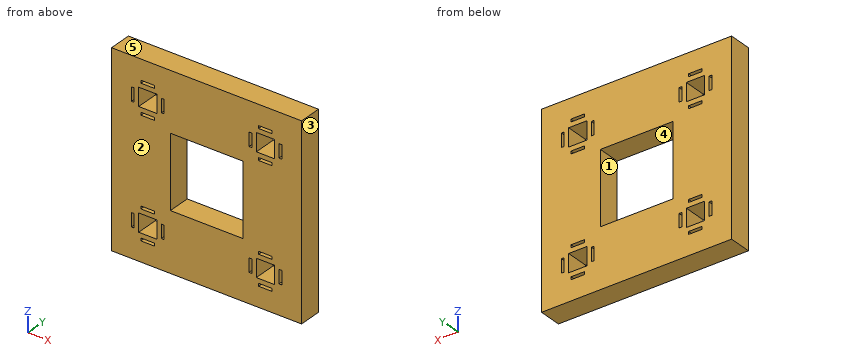
Autodesk Inventor part; units mm, degrees
ref_plane "YZ Plane" through (0, 0, 0) normal (1, 0, 0) x (0, 1, 0)
ref_plane "XZ Plane" through (0, 0, 0) normal (0, 1, 0) x (-1, 0, 0)
ref_plane "XY Plane" through (0, 0, 0) normal (0, 0, 1) x (1, 0, 0)
sketch "Sketch1" plane through (0, 0, 0) normal (0, 0, 1) x (1, 0, 0)
  line L0 (-105, 12.5) -> (105, 12.5)
  line L1 (105, 12.5) -> (105, -12.5)
  line L2 (105, -12.5) -> (-105, -12.5)
  line L3 (-105, -12.5) -> (-105, 12.5)
  line L4 (-105, 12.5) -> (105, -12.5) construction
  line L5 (105, 12.5) -> (-105, -12.5) construction
  point P0 (0, 0)
  dimension "d0" = 210
  dimension "d1" = 25
extrude "Extrusion1" add sketch "Sketch1" along normal mid plane 210
sketch "Sketch2" plane through (-105, -12.5, 105) normal (0, -1, 0) x (1, 0, 0)
  line L0 (0, -210) -> (0, 0)
  line L1 (0, -40) -> (210, -40)
  line L2 (210, -210) -> (210, 0)
  line L3 (0, -170) -> (210, -170)
  line L4 (0, -105) -> (210, -105)
  line L5 (0, 0) -> (210, 0)
  line L6 (105, 0) -> (105, -210)
  line L7 (170, 0) -> (170, -210)
  line L8 (40, 0) -> (40, -210)
  line L9 (210, -210) -> (0, -210)
  line L10 (0, 0) -> (0, -210)
  line L11 (162.5, -21.92) -> (177.5, -21.92)
  line L12 (177.5, -21.92) -> (177.5, -25)
  line L13 (177.5, -25) -> (162.5, -25)
  line L14 (162.5, -25) -> (162.5, -21.92)
  line L15 (162.5, -21.92) -> (177.5, -25) construction
  line L16 (177.5, -21.92) -> (162.5, -25) construction
  line L17 (188.08, -32.5) -> (185, -32.5)
  line L18 (185, -32.5) -> (185, -47.5)
  line L19 (185, -47.5) -> (188.08, -47.5)
  line L20 (188.08, -47.5) -> (188.08, -32.5)
  line L21 (188.08, -32.5) -> (185, -47.5) construction
  line L22 (185, -32.5) -> (188.08, -47.5) construction
  line L23 (162.5, -58.08) -> (177.5, -58.08)
  line L24 (177.5, -58.08) -> (177.5, -55)
  line L25 (177.5, -55) -> (162.5, -55)
  line L26 (162.5, -55) -> (162.5, -58.08)
  line L27 (162.5, -58.08) -> (177.5, -55) construction
  line L28 (177.5, -58.08) -> (162.5, -55) construction
  line L29 (188.08, -47.5) -> (185, -47.5)
  line L30 (185, -47.5) -> (185, -32.5)
  line L31 (185, -32.5) -> (188.08, -32.5)
  line L32 (188.08, -32.5) -> (188.08, -47.5)
  line L33 (188.08, -47.5) -> (185, -32.5) construction
  line L34 (185, -47.5) -> (188.08, -32.5) construction
  line L35 (151.92, -32.5) -> (155, -32.5)
  line L36 (155, -32.5) -> (155, -47.5)
  line L37 (155, -47.5) -> (151.92, -47.5)
  line L38 (151.92, -47.5) -> (151.92, -32.5)
  line L39 (151.92, -32.5) -> (155, -47.5) construction
  line L40 (155, -32.5) -> (151.92, -47.5) construction
  line L41 (155, -32.5) -> (151.92, -32.5)
  line L42 (155, -47.5) -> (155, -32.5)
  line L43 (151.92, -32.5) -> (151.92, -47.5)
  line L44 (155, -47.5) -> (151.92, -32.5) construction
  line L45 (151.92, -47.5) -> (155, -47.5)
  line L46 (151.92, -47.5) -> (155, -32.5) construction
  line L47 (47.5, -21.92) -> (32.5, -21.92)
  line L48 (32.5, -21.92) -> (32.5, -25)
  line L49 (32.5, -25) -> (47.5, -25)
  line L50 (47.5, -25) -> (47.5, -21.92)
  line L51 (47.5, -21.92) -> (32.5, -25) construction
  line L52 (32.5, -21.92) -> (47.5, -25) construction
  line L53 (21.92, -32.5) -> (25, -32.5)
  line L54 (25, -32.5) -> (25, -47.5)
  line L55 (25, -47.5) -> (21.92, -47.5)
  line L56 (21.92, -47.5) -> (21.92, -32.5)
  line L57 (21.92, -32.5) -> (25, -47.5) construction
  line L58 (25, -32.5) -> (21.92, -47.5) construction
  line L59 (32.5, -55) -> (47.5, -55)
  line L60 (47.5, -58.08) -> (32.5, -58.08)
  line L61 (32.5, -58.08) -> (47.5, -55) construction
  line L62 (47.5, -58.08) -> (32.5, -55) construction
  line L63 (47.5, -55) -> (47.5, -58.08)
  line L64 (32.5, -58.08) -> (32.5, -55)
  line L65 (25, -32.5) -> (21.92, -32.5)
  line L66 (25, -47.5) -> (25, -32.5)
  line L67 (21.92, -32.5) -> (21.92, -47.5)
  line L68 (25, -47.5) -> (21.92, -32.5) construction
  line L69 (21.92, -47.5) -> (25, -47.5)
  line L70 (21.92, -47.5) -> (25, -32.5) construction
  line L71 (55, -32.5) -> (58.08, -32.5)
  line L72 (58.08, -32.5) -> (55, -32.5)
  line L73 (55, -47.5) -> (55, -32.5)
  line L74 (55, -32.5) -> (55, -47.5)
  line L75 (58.08, -47.5) -> (55, -47.5)
  line L76 (58.08, -32.5) -> (58.08, -47.5)
  line L77 (55, -47.5) -> (58.08, -32.5) construction
  line L78 (58.08, -47.5) -> (55, -32.5) construction
  line L79 (55, -47.5) -> (58.08, -47.5)
  line L80 (58.08, -47.5) -> (58.08, -32.5)
  line L81 (55, -32.5) -> (58.08, -47.5) construction
  line L82 (58.08, -32.5) -> (55, -47.5) construction
  line L83 (162.5, -188.08) -> (177.5, -188.08)
  line L84 (177.5, -188.08) -> (177.5, -185)
  line L85 (177.5, -185) -> (162.5, -185)
  line L86 (162.5, -185) -> (162.5, -188.08)
  line L87 (162.5, -188.08) -> (177.5, -185) construction
  line L88 (177.5, -188.08) -> (162.5, -185) construction
  line L89 (188.08, -177.5) -> (185, -177.5)
  line L90 (185, -177.5) -> (185, -162.5)
  line L91 (185, -162.5) -> (188.08, -162.5)
  line L92 (188.08, -162.5) -> (188.08, -177.5)
  line L93 (188.08, -177.5) -> (185, -162.5) construction
  line L94 (185, -177.5) -> (188.08, -162.5) construction
  line L95 (177.5, -155) -> (162.5, -155)
  line L96 (162.5, -151.92) -> (177.5, -151.92)
  line L97 (177.5, -151.92) -> (162.5, -155) construction
  line L98 (162.5, -151.92) -> (177.5, -155) construction
  line L99 (162.5, -155) -> (162.5, -151.92)
  line L100 (177.5, -151.92) -> (177.5, -155)
  line L101 (185, -177.5) -> (188.08, -177.5)
  line L102 (185, -162.5) -> (185, -177.5)
  line L103 (188.08, -177.5) -> (188.08, -162.5)
  line L104 (185, -162.5) -> (188.08, -177.5) construction
  line L105 (188.08, -162.5) -> (185, -162.5)
  line L106 (188.08, -162.5) -> (185, -177.5) construction
  line L107 (155, -177.5) -> (151.92, -177.5)
  line L108 (151.92, -177.5) -> (155, -177.5)
  line L109 (155, -162.5) -> (155, -177.5)
  line L110 (155, -177.5) -> (155, -162.5)
  line L111 (151.92, -162.5) -> (155, -162.5)
  line L112 (151.92, -177.5) -> (151.92, -162.5)
  line L113 (155, -162.5) -> (151.92, -177.5) construction
  line L114 (151.92, -162.5) -> (155, -177.5) construction
  line L115 (155, -162.5) -> (151.92, -162.5)
  line L116 (151.92, -162.5) -> (151.92, -177.5)
  line L117 (155, -177.5) -> (151.92, -162.5) construction
  line L118 (151.92, -177.5) -> (155, -162.5) construction
  line L119 (55, -177.5) -> (58.08, -177.5)
  line L120 (58.08, -177.5) -> (58.08, -162.5)
  line L121 (55, -162.5) -> (58.08, -177.5) construction
  line L122 (58.08, -162.5) -> (55, -177.5) construction
  line L123 (58.08, -177.5) -> (55, -177.5)
  line L124 (58.08, -162.5) -> (58.08, -177.5)
  line L125 (55, -177.5) -> (58.08, -162.5) construction
  line L126 (58.08, -177.5) -> (55, -162.5) construction
  line L127 (58.08, -162.5) -> (55, -162.5)
  line L128 (55, -162.5) -> (58.08, -162.5)
  line L129 (25, -162.5) -> (21.92, -162.5)
  line L130 (21.92, -162.5) -> (25, -162.5)
  line L131 (25, -177.5) -> (25, -162.5)
  line L132 (25, -162.5) -> (25, -177.5)
  line L133 (21.92, -162.5) -> (21.92, -177.5)
  line L134 (25, -177.5) -> (21.92, -162.5) construction
  line L135 (21.92, -177.5) -> (25, -162.5) construction
  line L136 (21.92, -177.5) -> (25, -177.5)
  line L137 (21.92, -162.5) -> (25, -177.5) construction
  line L138 (21.92, -177.5) -> (21.92, -162.5)
  line L139 (25, -177.5) -> (21.92, -177.5)
  line L140 (25, -162.5) -> (21.92, -177.5) construction
  line L141 (47.5, -188.08) -> (32.5, -188.08)
  line L142 (32.5, -188.08) -> (32.5, -185)
  line L143 (32.5, -185) -> (47.5, -185)
  line L144 (47.5, -185) -> (47.5, -188.08)
  line L145 (47.5, -188.08) -> (32.5, -185) construction
  line L146 (32.5, -188.08) -> (47.5, -185) construction
  line L147 (55, -162.5) -> (55, -177.5)
  line L148 (55, -177.5) -> (55, -162.5)
  line L149 (32.5, -151.92) -> (32.5, -155)
  line L150 (32.5, -155) -> (47.5, -155)
  line L151 (32.5, -151.92) -> (47.5, -155) construction
  line L152 (47.5, -151.92) -> (32.5, -155) construction
  line L153 (47.5, -155) -> (47.5, -151.92)
  line L154 (47.5, -151.92) -> (32.5, -151.92)
  line L155 (160, -30) -> (180, -30)
  line L156 (180, -30) -> (180, -50)
  line L157 (180, -50) -> (160, -50)
  line L158 (160, -50) -> (160, -30)
  line L159 (160, -30) -> (180, -50) construction
  line L160 (180, -30) -> (160, -50) construction
  line L161 (30, -50) -> (50, -50)
  line L162 (50, -50) -> (50, -30)
  line L163 (50, -30) -> (30, -30)
  line L164 (30, -30) -> (30, -50)
  line L165 (30, -50) -> (50, -30) construction
  line L166 (50, -50) -> (30, -30) construction
  line L167 (30, -160) -> (50, -160)
  line L168 (50, -160) -> (50, -180)
  line L169 (50, -180) -> (30, -180)
  line L170 (30, -180) -> (30, -160)
  line L171 (30, -160) -> (50, -180) construction
  line L172 (50, -160) -> (30, -180) construction
  line L173 (160, -160) -> (180, -160)
  line L174 (180, -160) -> (180, -180)
  line L175 (180, -180) -> (160, -180)
  line L176 (160, -180) -> (160, -160)
  line L177 (160, -160) -> (180, -180) construction
  line L178 (180, -160) -> (160, -180) construction
  point P0 (105, -105)
  point P1 (170, -23.46)
  point P2 (186.54, -40)
  point P3 (170, -56.54)
  point P4 (153.46, -40)
  point P5 (40, -23.46)
  point P6 (23.46, -40)
  point P7 (40, -56.54)
  point P8 (56.54, -40)
  point P9 (170, -186.54)
  point P10 (186.54, -170)
  point P11 (170, -153.46)
  point P12 (153.46, -170)
  point P13 (56.54, -170)
  point P14 (23.46, -170)
  point P15 (40, -186.54)
  point P16 (40, -153.46)
  point P17 (170, -40)
  point P18 (40, -40)
  point P19 (40, -170)
  point P20 (170, -170)
  dimension "d4" = 40
  dimension "d5" = 40
  dimension "d8" = 15
  dimension "d9" = 3.08
  dimension "d10" = 30
  dimension "d11" = 15
  dimension "d12" = 30
  dimension "d13" = 3.08
  dimension "d20" = 20
  dimension "d21" = 20
  dimension "d22" = 20
  dimension "d23" = 20
  dimension "d24" = 20
  dimension "d25" = 20
  dimension "d26" = 20
  dimension "d27" = 20
extrude "Extrusion2" cut sketch "Sketch2" against normal through all contours L133 L129 L131 L3 | L3 L131 L136 L133 | L141 L142 L143 L8 | L8 L143 L144 L141 | L56 L53 L54 L1 | L1 L54 L55 L56 | L60 L64 L59 L8 | L8 L59 L63 L60 | L154 L153 L150 L8 | L8 L150 L149 L154 | L170 L167 L8 L3 | L3 L8 L169 L170 | L8 L3 L168 L169 | L120 L119 L147 L3 | L3 L147 L127 L120 | L112 L111 L109 L3 | L3 L109 L107 L112 | L83 L86 L85 L7 | L7 L85 L84 L83 | L8 L167 L168 L3 | L47 L50 L49 L8 | L8 L49 L48 L47 | L164 L163 L8 L1 | L1 L8 L161 L164 | L23 L26 L25 L7 | L7 L25 L24 L23 | L96 L100 L95 L7 | L7 L95 L99 L96 | L76 L75 L73 L1 | L1 L73 L71 L76 | L38 L35 L36 L1 | L1 L36 L37 L38 | L8 L1 L162 L161 | L176 L173 L7 L3 | L3 L7 L175 L176 | L7 L3 L174 L175 | L92 L89 L90 L3 | L3 L90 L91 L92 | L8 L163 L162 L1 | L7 L173 L174 L3 | L11 L12 L13 L7 | L7 L13 L14 L11 | L20 L19 L18 L1 | L1 L18 L17 L20 | L157 L158 L1 L7 | L7 L1 L156 L157 | L158 L155 L7 L1 | L7 L155 L156 L1
sketch "Sketch3" plane through (-105, 12.5, 105) normal (0, 1, 0) x (1, 0, 0)
  line L0 (65, 65) -> (145, 65)
  line L1 (145, 65) -> (145, 145)
  line L2 (145, 145) -> (65, 145)
  line L3 (65, 145) -> (65, 65)
  line L4 (65, 65) -> (145, 145) construction
  line L5 (145, 65) -> (65, 145) construction
  point P0 (105, 105)
  dimension "d16" = 80
  dimension "d17" = 80
extrude "Extrusion3" cut sketch "Sketch3" against normal through all
equation "\"d5\" = d4"
equation "\"d12\" = d10"
equation "\"d13\" = d9"
properties part number "Box Of Fixation"
Geometry check sheet. Reference: the model listing, model coordinates, mm. Face numbers are marked on the shaded views. A direction names the side the tool comes from. Give positions to 0.01 mm unless a question says otherwise; leave off trailing zeros. Loops run counter-clockwise (first coordinate to the right, second up) from the corner with the lowest first, then second, coordinate; pieces in that order, holes last. Notation, with made-up numbers: M 72.25,64 L 129.25,64 A4 cw 129.25,68 Z; hole C -21,43 d9. An arc over 180 degrees is marked long. Answer as CSV lines item,"result".
Item 1: Cross-section at C-C on z = 63.5. Record the cut outline in (x, y), and give its area (3 significant figures).
Values:
outline,"M -105,-12.5 L -83.08,-12.5 L -83.08,12.5 L -105,12.5 Z; M -80,-12.5 L -75,-12.5 L -75,12.5 L -80,12.5 Z; M -55,-12.5 L -50,-12.5 L -50,12.5 L -55,12.5 Z; M -46.92,-12.5 L 46.92,-12.5 L 46.92,12.5 L -46.92,12.5 Z; M 50,-12.5 L 55,-12.5 L 55,12.5 L 50,12.5 Z; M 75,-12.5 L 80,-12.5 L 80,12.5 L 75,12.5 Z; M 83.08,-12.5 L 105,-12.5 L 105,12.5 L 83.08,12.5 Z"
area,"3,940 mm²"
Item 2: Material ranges on line 1 (Z direction, x = -83, y = -9.75); line 2 (Z direction, x = 1, y = -2.5), recorded low to high.
Values:
line 1,"z = -105 to -72.5, -57.5 to 57.5, 72.5 to 105"
line 2,"z = -105 to -40, 40 to 105"
Item 3: Release check for a two-part mould opening along X. For the marked faces 1, 2 and 3 record: pulls with the +X half, pulls with the -X half, needs draft (parallel to the pull), parting line crosses it, or undercut.
Values:
face 1,"undercut"
face 2,"needs draft"
face 3,"pulls with the +X half"
Item 4: Cross-section at D-D on y = 0.75. Count the separate pieces of the cut face and the enclosed holes in it, and give its area (3 significant figures).
Values:
separate pieces,"1"
enclosed holes,"21"
area,"35,400 mm²"
Item 5: Access from +Z, -Z, +X, -X, +Y, -Y to the whole of each face (thin tool, end or side, straight path). Record for the marked faces 4 and 5.
Values:
face 4,"+Y, -Y"
face 5,"+Z, +X, -X, +Y, -Y"
Item 6: Depth check by flat-ended pin: P1, Ø1, axis at x = 49, z = 62.5, coming from the +Y side. Enter the tip coordinate at first touch or a pass-through.
Values:
P1,"passes through"
Item 7: Cross-section at B-B on z = 27.5. Record the cut outline in (x, y).
Values:
outline,"M -105,-12.5 L -40,-12.5 L -40,12.5 L -105,12.5 Z; M 40,-12.5 L 105,-12.5 L 105,12.5 L 40,12.5 Z"
Item 8: Cross-section at A-A on x = -61. Record the cut outline in (y, z), and give its area (3 significant figures).
Values:
outline,"M -12.5,-105 L 12.5,-105 L 12.5,-83.08 L -12.5,-83.08 Z; M -12.5,-80 L 12.5,-80 L 12.5,-75 L -12.5,-75 Z; M -12.5,-55 L 12.5,-55 L 12.5,-50 L -12.5,-50 Z; M -12.5,-46.92 L 12.5,-46.92 L 12.5,46.92 L -12.5,46.92 Z; M -12.5,50 L 12.5,50 L 12.5,55 L -12.5,55 Z; M -12.5,75 L 12.5,75 L 12.5,80 L -12.5,80 Z; M -12.5,83.08 L 12.5,83.08 L 12.5,105 L -12.5,105 Z"
area,"3,940 mm²"
